```python
from build123d import *

# Parameters (mm, degrees)
SKETCH1_W           = 20
SKETCH1_H           = 15
BOSS_EXTRUDE1_DEPTH = 5
SKETCH2_R           = 2.5
CUT_EXTRUDE1_DEPTH  = 5
SKETCH3_W           = 3
SKETCH3_H           = 15
BOSS_EXTRUDE2_DEPTH = 40
SKETCH5_W           = 2.5
SKETCH5_H           = 12.5
CUT_EXTRUDE3_DEPTH  = 6
SKETCH4_R           = 2.5
CUT_EXTRUDE4_DEPTH  = 10


with BuildPart() as part:
    # Sketch1 → Boss-Extrude1 (new body)
    with BuildSketch(Plane.XY):
        with Locations((10, 7.5)):
            Rectangle(SKETCH1_W, SKETCH1_H)
    extrude(amount=BOSS_EXTRUDE1_DEPTH)

    # Sketch2 → Cut-Extrude1 (cut)
    with BuildSketch(Plane.XY.offset(5)):
        with Locations((7.5, 7.5)):
            Circle(SKETCH2_R)
    extrude(amount=-CUT_EXTRUDE1_DEPTH, mode=Mode.SUBTRACT)

    # Sketch3 → Boss-Extrude2 (add)
    with BuildSketch(Plane(origin=(0, 0, 0), x_dir=(-1, 0, 0), z_dir=(0, 0, -1))):
        with Locations((-13.5, 7.5)):
            Rectangle(SKETCH3_W, SKETCH3_H)
    extrude(amount=BOSS_EXTRUDE2_DEPTH)

    # Sketch5 → Cut-Extrude3 (cut, through all)
    with BuildSketch(Plane(origin=(0, 0, 0), x_dir=(-1, 0, 0), z_dir=(0, 0, -1))):
        with Locations((-17.5, 7.5)):
            Rectangle(SKETCH5_W, SKETCH5_H)
    extrude(amount=-CUT_EXTRUDE3_DEPTH, mode=Mode.SUBTRACT)

    # Sketch4 → Cut-Extrude4 (cut)
    with BuildSketch(Plane(origin=(15, 0, 0), x_dir=(0, 0, -1), z_dir=(1, 0, 0))):
        with Locations((35, 7.5)):
            Circle(SKETCH4_R)
    extrude(amount=-CUT_EXTRUDE4_DEPTH, mode=Mode.SUBTRACT)


solid = part.part
```
Can you work these out from the model? Positions are in its coordinate system, mm. A direction names the side the tool comes from. Round coordinates to 2 decimals unless told otherwise and drop trailing zeros. Loops run counter-clockwise (first coordinate to the right, second up) from the corner with the lowest first, then second, coordinate; pieces in that order, holes last. Notation, with made-up numbers: M 60.5,67.5 L 118.5,67.5 A18 ccw 118.5,99.5 Z; hole C -12,26.25 d2. An arc over 180 degrees is marked long. Write item = value, one per line. Start each with the question number.
(1) Which directions (+Z, -Z, +X, -X, +Y, -Y) give clear straight access to the entire face, cutting with the end or side of a thin tool? Please do faces 5 (the face through (16, 8, 0)), 6 (the face through (13, 15, -9)), 7 (the face through (18, 1.25, 2)), 8 (the face through (14, 8, -40)), 9 (the face through (12, 7, -20)).
(2) I need wall thicknesses on line 1 along Y through (x, z) = (7.5, 3.8); line 2 along Y through (x, z) = (17.75, 3.5); line 3 along X through (y, z) = (14.75, -24.5). Which ranges of each line are inside material? Lowest first, please.
(3) I'm going to push flat-ended pins straight in: P1, Ø8, axis at x = 7.5, y = 7.5, coming from the -Z side; P2, Ø4, axis at y = 7.5, z = -35, coming from the +X side. Where does each tip first touch, or does it pass through?
(4) Suppose I cut it at D-D on y = 1.75. Write out the boundary of the cut face in (x, z), plus the area to 4 significant figures.
(5) Suppose I cut it at C-C on z = -35. Write out the boundary of the cut face in (x, y).
(6) Suppose I cut it at B-B on x = 7.5. Write out the boundary of the cut face in (y, z).
(7) If we mould it in two halves opening along X, with no side actions, what happens to faces 1 (the face through (15, 7, -20)), 2 (the face through (8.65, 5.28, 2.54)), 3 (the face through (4.6, 7.6, 0)), 4 (the face through (16.25, 7, 2))? For each: released by +X, released by -X, zero draft, split by the parting line, or undercut.
(8) Suppose I cut it at A-A on y = 6. Write out the boundary of the cut face in (x, z), plus the area to 4 significant figures.
Answer block:
q1.face_5 = -Z, +X, +Y, -Y
q1.face_6 = +Z, -Z, +X, -X, +Y
q1.face_7 = +Z, -Z
q1.face_8 = -Z, +X, -X, +Y, -Y
q1.face_9 = -Z, -X, +Y, -Y
q2.line_1 = 0 to 5, 10 to 15
q2.line_2 = 0 to 1.25, 13.75 to 15
q2.line_3 = 12 to 15
q3.P1 = 0
q3.P2 = through
q4.outline = M 0,0 L 12,0 L 12,-40 L 15,-40 L 15,0 L 16.25,0 L 16.25,5 L 0,5 Z; M 18.75,0 L 20,0 L 20,5 L 18.75,5 Z
q4.area = 207.5 mm²
q5.outline = M 12,0 L 15,0 L 15,5 L 12,5 Z; M 12,10 L 15,10 L 15,15 L 12,15 Z
q6.outline = M 0,0 L 5,0 L 5,5 L 0,5 Z; M 10,0 L 15,0 L 15,5 L 10,5 Z
q7.face_1 = released by +X
q7.face_2 = undercut
q7.face_3 = zero draft
q7.face_4 = undercut
q8.outline = M 0,0 L 5.5,0 L 5.5,5 L 0,5 Z; M 9.5,0 L 12,0 L 12,-33 L 15,-33 L 15,0 L 16.25,0 L 16.25,5 L 9.5,5 Z; M 12,-40 L 15,-40 L 15,-37 L 12,-37 Z; M 18.75,0 L 20,0 L 20,5 L 18.75,5 Z
q8.area = 175.5 mm²
